The model under review builds one solid part; all positions refer to its coordinate system, in mm. Face numbers are marked on the shaded views. A direction names the side the tool comes from. Coordinates: 2 decimals unless noted, no trailing zeros. Loops run counter-clockwise (first coordinate to the right, second up) from the corner with the lowest first, then second, coordinate; pieces in that order, holes last. Notation, with made-up numbers: (45, 11) - (74, 11) arc R25 cw to (74, 40) - close; hole circle Ø10 at (4.5, -1). An arc over 180 degrees is marked (long way). Answer in a Markdown table with one row per item. Add a question column.
(1) Machinability: for the marked faces 1 and 2, which of the approach directions +Z, -Z, +X, -X, +Y, -Y give a long, thin tool a straight path to every point of the face, cutting with its end or side? Answer none if there is none.
(2) We need section C-C on y = -1.5. Write out the cut boundary in (x, z) (3 decimals).
(3) We need section B-B on y = 0.5. Write out the cut boundary in (x, z).
(4) We need section A-A on y = 4. Write out the cut boundary in (x, z) (3 decimals).
(5) For line 1 along X through (y, z) = (1, 11.5); line 2 along Y through (x, z) = (18.75, 12.75); line 3 along Y through (x, z) = (24.25, 11), list the stretches that pass through material, from the lowest coordinate up.
(6) For P1, Ø6, axis at y = -2, z = 14, coming from the +X side; P2, Ø0.8, axis at y = 0.5, z = 19.5, coming from the -X side; P3, Ø0.8, axis at x = 22.5, z = 13.5, coming from the -Y side; P4, Ø0.8, axis at y = 0.5, z = 19.5, coming from the +X side, all flat-tipped, find the tip position at first contact; note any pin that passes through.
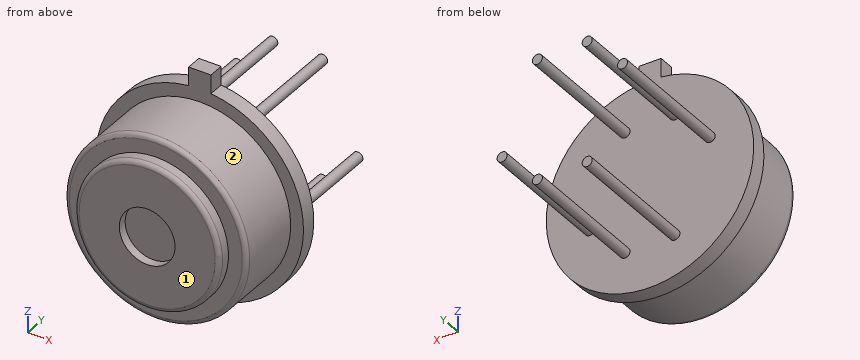
from build123d import *

# Parameters (mm, degrees)
SKETCH1_R           = 4.65
BOSS_EXTRUDE1_DEPTH = 0.7
SKETCH2_R           = 4.075
BOSS_EXTRUDE2_DEPTH = 3
SKETCH3_R           = 3.25
BOSS_EXTRUDE3_DEPTH = 0.6
FILLET1_R           = 0.2
FILLET2_R           = 0.2
SKETCH4_R           = 1.25
CUT_EXTRUDE1_DEPTH  = 0.4
SKETCH5_W           = 1
SKETCH5_H           = 1.626707286
BOSS_EXTRUDE4_DEPTH = 0.7
SKETCH6_R           = 0.225
BOSS_EXTRUDE5_DEPTH = 6


with BuildPart() as part:
    # Sketch1 → Boss-Extrude1 (new body)
    with BuildSketch(Plane(origin=(0, 0, 0), x_dir=(1, 0, 0), z_dir=(0, 1, 0))):
        with Locations(Location((22.683106859, -14.228561536, 0), (0, 0, 270))):
            Circle(SKETCH1_R)
    extrude(amount=BOSS_EXTRUDE1_DEPTH)

    # Sketch2 → Boss-Extrude2 (add)
    with BuildSketch(Plane.XZ):
        with Locations(Location((22.683106859, 14.228561536, 0), (0, 0, 270))):
            Circle(SKETCH2_R)
    extrude(amount=BOSS_EXTRUDE2_DEPTH)

    # Sketch3 → Boss-Extrude3 (add)
    with BuildSketch(Plane.XZ.offset(3)):
        with Locations(Location((22.683106859, 14.228561536, 0), (0, 0, 270))):
            Circle(SKETCH3_R)
    extrude(amount=BOSS_EXTRUDE3_DEPTH)

    # Fillet1
    fillet1_edges = [part.edges().sort_by_distance(p)[0] for p in [
        (22.683106859, -3, 18.303561536),
    ]]
    fillet(fillet1_edges, radius=FILLET1_R)

    # Fillet2
    fillet2_edges = [part.edges().sort_by_distance(p)[0] for p in [
        (22.683106859, -3.6, 17.478561536),
    ]]
    fillet(fillet2_edges, radius=FILLET2_R)

    # Sketch4 → Cut-Extrude1 (cut)
    with BuildSketch(Plane.XZ.offset(3.6)):
        with Locations(Location((22.683106859, 14.228561536, 0), (0, 0, 270))):
            Circle(SKETCH4_R)
    extrude(amount=-CUT_EXTRUDE1_DEPTH, mode=Mode.SUBTRACT)

    # Sketch5 → Boss-Extrude4 (add)
    with BuildSketch(Plane(origin=(0, 0.7, 0), x_dir=(1, 0, 0), z_dir=(0, 1, 0))):
        with Locations((22.683106859, -18.875207893)):
            Rectangle(SKETCH5_W, SKETCH5_H)
    extrude(amount=-BOSS_EXTRUDE4_DEPTH)

    # Sketch6 → Boss-Extrude5 (add)
    with BuildSketch(Plane(origin=(0, 0.7, 0), x_dir=(1, 0, 0), z_dir=(0, 1, 0))):
        with Locations(Location((19.985378624, -15.345997158, 0), (0, 0, 270))):
            Circle(SKETCH6_R)
        with Locations(Location((21.565671236, -16.926289771, 0), (0, 0, 270))):
            Circle(SKETCH6_R)
        with Locations(Location((23.800542481, -16.926289771, 0), (0, 0, 270))):
            Circle(SKETCH6_R)
        with Locations(Location((25.380835094, -13.111125913, 0), (0, 0, 270))):
            Circle(SKETCH6_R)
        with Locations(Location((23.800542481, -11.530833301, 0), (0, 0, 270))):
            Circle(SKETCH6_R)
        with Locations(Location((21.565671236, -11.530833301, 0), (0, 0, 270))):
            Circle(SKETCH6_R)
    extrude(amount=BOSS_EXTRUDE5_DEPTH)


solid = part.part
Outcome:
| question | item | result |
|---|---|---|
| 1 | face 1 | +Z, -Z, +X, -X, -Y |
| 1 | face 2 | -Y |
| 2 | outline | circle Ø8.15 at (22.683, 14.229) |
| 3 | outline | (22.18, 18.85) arc R4.65 ccw (long way) to (23.18, 18.85) - (23.18, 19.69) - (22.18, 19.69) - close |
| 4 | outline | circle Ø0.45 at (19.985, 15.346); circle Ø0.45 at (21.566, 11.531); circle Ø0.45 at (21.566, 16.926); circle Ø0.45 at (23.801, 11.531); circle Ø0.45 at (23.801, 16.926); circle Ø0.45 at (25.381, 13.111) |
| 5 | line 1 | 21.34 to 21.79, 23.58 to 24.02 |
| 5 | line 2 | 0 to 0.7 |
| 5 | line 3 | -3 to 0.7 |
| 6 | P1 | x = 27.33 |
| 6 | P2 | x = 22.18 |
| 6 | P3 | y = -3.2 |
| 6 | P4 | x = 23.18 |
